Verification items for the finished model (mm, model axes). A direction names the side the tool comes from. Round coordinates to 2 decimals unless told otherwise and drop trailing zeros. Loops run counter-clockwise (first coordinate to the right, second up) from the corner with the lowest first, then second, coordinate; pieces in that order, holes last. Notation, with made-up numbers: (25.5, 41.25) -> (41.5, 41.25) arc R27 cw to (41.5, 67.25) -> close; hole circle Ø4 at (-31, 64.25). An arc over 180 degrees is marked (long way). Write item = value, one per line. Start each with the question number.
```python
from build123d import *

# Parameters (mm, degrees)
F0_R     = 15
F1_DEPTH = 75
F2_R     = 10
F3_DEPTH = 10
F4_R     = 5
F5_DEPTH = 15


with BuildPart() as f1:
    # F0 (on Front) → F1 (new body)
    with BuildSketch(Plane.XZ):
        with BuildLine():
            Line((-88.529155, 50), (-88.529155, -25))
            Line((-88.529155, -25), (-38.529155, -25))
            ThreePointArc((-38.529155, -25), (-20.851485, -17.67767), (-13.529155, 0))
            Line((-13.529155, 0), (-13.529155, 10))
            Line((-13.529155, 10), (31.470845, 10))
            Line((31.470845, 10), (31.470845, 25))
            Line((31.470845, 25), (-38.529155, 25))
            ThreePointArc((-38.529155, 25), (-56.206824, 17.67767), (-63.529155, 0))
            Line((-63.529155, 0), (-63.529155, -10))
            Line((-63.529155, -10), (-78.529155, -10))
            Line((-78.529155, -10), (-78.529155, 50))
            Line((-78.529155, 50), (-88.529155, 50))
        make_face()
        with Locations((-38.529155, 0)):
            Circle(F0_R, mode=Mode.SUBTRACT)
    extrude(amount=F1_DEPTH)

    # F2 (on face) → F3 (cut)
    with BuildSketch(Plane(origin=(-88.529155, 0, 0), x_dir=(0, -1, 0), z_dir=(-1, 0, 0))):
        Polygon((0, 35), (15, 50), (0, 50), align=None)
        Polygon((75, 50), (60, 50), (75, 35), align=None)
        with Locations((35, 15)):
            Circle(F2_R)
    extrude(amount=-F3_DEPTH, mode=Mode.SUBTRACT)

    # F4 (on face) → F5 (cut)
    with BuildSketch(Plane.XY.offset(25)):
        with Locations((16.470845, -20)):
            Circle(F4_R)
        with Locations((16.470845, -55)):
            Circle(F4_R)
    extrude(amount=-F5_DEPTH, mode=Mode.SUBTRACT)


solid = f1.part
```
(1) Draft check along Y on faces 4 (the cylindrical face through (15.82, -50.043, 17.605)), 5 (the flat face through (-56, 0, 5)), 6 (the cylindrical face through (-41.781, -36.975, -14.643)). Enter one of: +Y half, -Y half, draft (parallel to the pull), parting line (faces both ways), or undercut.
(2) Section check C-C on x = -40.5. Enter the section's corners in (y, z).
(3) Depth check by flat-ended pin: pin 1 Ø4.5 at (x, y) = (-69.5, -19.5) entering from +Z; pin 2 Ø22.5 at (x, y) = (-0.5, -19) entering from -Z; pin 3 Ø1 at (x, y) = (-28.5, -34.5) entering from -Z; pin 4 Ø9 at (x, y) = (16.47, -55) entering from -Z. Enter the tip coordinate at first touch or a pass-through.
(4) Section check A-A on y = -35. Enter the section's corners in (x, z), then the cut area to 3 significant figures.
(5) Section check D-D on z = -11.5. Enter the section's corners in (x, y).
(6) Access from +Z, -Z, +X, -X, +Y, -Y to the whole of each face (thin tool, end or side, straight path). Record for faces 1 (the cylindrical face through (-56.01, -36.98, 17.87)), 2 (the flat face through (-13.529, -37, 5)), 3 (the flat face through (-3, -37, 25)).
(7) Scan lines: line 1 (X direction, y = -28, z = -3); line 2 (Z direction, x = -81.25, y = -35); line 3 (X direction, y = -44.5, z = -8). Record each from-to range of solid material in increasing order. Write a range as [from, to].
(8) Section check B-B on y = -63. Enter the section's corners in (x, z).
Computed values:
q1.face_4 = undercut
q1.face_5 = +Y half
q1.face_6 = draft
q2.outline = (-75, -25) -> (0, -25) -> (0, -14.87) -> (-75, -14.87) -> close; (-75, 14.87) -> (0, 14.87) -> (0, 24.92) -> (-75, 24.92) -> close
q3.pin_1 = -10
q3.pin_2 = 10
q3.pin_3 = -23.11
q3.pin_4 = through
q4.outline = (-88.53, -25) -> (-38.53, -25) arc R25 ccw to (-13.53, 0) -> (-13.53, 10) -> (31.47, 10) -> (31.47, 25) -> (-38.53, 25) arc R25 ccw to (-63.53, 0) -> (-63.53, -10) -> (-78.53, -10) -> (-78.53, 5) -> (-88.53, 5) -> close; (-88.53, 25) -> (-78.53, 25) -> (-78.53, 50) -> (-88.53, 50) -> close; hole circle Ø30 at (-38.53, 0)
q4.area = 2,970 mm²
q5.outline = (-88.53, -75) -> (-48.16, -75) -> (-48.16, 0) -> (-88.53, 0) -> close; (-28.9, -75) -> (-16.33, -75) -> (-16.33, 0) -> (-28.9, 0) -> close
q6.face_1 = +Z, +Y, -Y
q6.face_2 = -Z, +X, +Y, -Y
q6.face_3 = +Z, +X, +Y, -Y
q7.line_1 = [-88.53, -78.53], [-63.53, -53.23], [-23.83, -13.71]
q7.line_2 = [-25, 5], [25, 50]
q7.line_3 = [-88.53, -78.53], [-63.53, -51.22], [-25.84, -14.84]
q8.outline = (-88.53, -25) -> (-38.53, -25) arc R25 ccw to (-13.53, 0) -> (-13.53, 10) -> (31.47, 10) -> (31.47, 25) -> (-38.53, 25) arc R25 ccw to (-63.53, 0) -> (-63.53, -10) -> (-78.53, -10) -> (-78.53, 47) -> (-88.53, 47) -> close; hole circle Ø30 at (-38.53, 0)
